Solid Edge part; units mm, degrees
sketch "Sketch1" plane through (0, 0, 0) normal (0, 0, -1) x (-1, 0, 0)
  circle A0 centre (5.5571, -5.7478) radius 2.6503
  line L0 (-56.7501, 0) -> (-56.7501, 10)
  line L1 (-56.7501, 10) -> (67.8618, 10)
  line L2 (67.8618, 0) -> (67.8618, 10)
  line L3 (37.8136, -15.4719) -> (67.8618, 0)
  line L4 (-26.5984, -15.5762) -> (37.8136, -15.4719)
  line L5 (-56.7501, 0) -> (-26.5984, -15.5762)
  circle A1 centre (-19.4469, -5.7778) radius 2.6727
  circle A2 centre (30.5773, -5.7557) radius 2.66
extrude "Protrusion1" add sketch "Sketch1" along normal blind 12
sketch "Sketch2" plane through (56.7501, 5, -6) normal (1, 0, 0) x (0, 0, 1)
  line L0 (-6, -14.1297) -> (-20, 5)
  line L1 (-20, 5) -> (-6, 20.5762)
  line L2 (-6, 20.5762) -> (3.5539, -5)
  line L3 (3.5539, -5) -> (-6, -14.1297)
extrude "ExtrudedCutout_2" cut sketch "Sketch2" along normal mid plane 258
sketch "Sketch3" plane through (0, 0, 0) normal (0, 0, -1) x (-1, 0, 0)
  line L0 (37.8136, -15.4719) -> (67.8618, 0)
  line L1 (67.8618, 0) -> (67.8618, 10)
  line L2 (-56.7501, 10) -> (67.8618, 10)
  line L3 (-56.7501, 0) -> (-56.7501, 10)
  line L4 (-56.7501, 0) -> (-26.5984, -15.5762)
  line L5 (-26.5984, -15.5762) -> (37.8136, -15.4719)
  circle A0 centre (30.5773, -5.7557) radius 2.66
  circle A1 centre (5.5571, -5.7478) radius 2.6503
  circle A2 centre (-19.4469, -5.7778) radius 2.6727
extrude "ExtrudedCutout_3" cut sketch "Sketch3" along normal blind 2.5
Design review of the part built by this model. Coordinates are the model's own, in mm. Coordinates: 2 decimals unless noted, no trailing zeros. Loops run counter-clockwise (first coordinate to the right, second up) from the corner with the lowest first, then second, coordinate; pieces in that order, holes last. Notation, with made-up numbers: (53.5, 41) -> (79.5, 41) arc R24 ccw to (79.5, 75) -> close; hole circle Ø3 at (11.25, -4). An arc over 180 degrees is marked (long way). Use a Markdown table: item, result. Add a question column.
Item 1: Wall thickness on L1, parallel to X at y = -8, z = -4; L2, parallel to Z at x = 31, y = -6; L3, parallel to X at y = -7.75, z = -5.25: over which ranges is each line inside the solid? List them lowest first. Write a range as from..to.
Item 2: We need section C-C, the plane y = -11.25. Write out the cut boundary in (x, z), and give its area (3 significant figures).
Item 3: We need section D-D, the plane z = -10.75. Write out the cut boundary in (x, y).
Item 4: The part is to be moulded in two halves that separate along X. For faces 1 (the flat face through (-5, 0, -2.5)), 2 (the flat face through (38.535, -9.41, -6.128)), 3 (the cylindrical face through (-30.231, -8.393, -5.108)), say which applies: +X half, -X half, draft (parallel to the pull), parting line (faces both ways), or undercut.
Item 5: We need section B-B, the plane z = -4.75. Write out the cut boundary in (x, y).
Item 6: Clearance check with flat-ended pins moving along their axes: P1, Ø10, axis at x = 22, y = 0.5, coming from the -Z side; P2, Ø8.5, axis at x = -5.56, y = -5.75, coming from the -Z side; P3, Ø4, axis at y = -12, z = -6, coming from the +X side. State where each tip first meets the part, or that it passes through.
Item 7: We need section A-A, the plane x = -31.5. Write out the cut boundary in (y, z).
Numbers:
| question | item | result |
|---|---|---|
| 1 | L1 | x = -52.32..-32.01, -29.15..-6.95, -4.16..17.96, 20.93..41.26 |
| 1 | L2 | z = -8.42..-2.5 |
| 1 | L3 | x = -52.81..-32.34, -28.82..-7.29, -3.82..17.64, 21.25..41.75 |
| 2 | outline | (-46.01, -10.38) -> (34.97, -10.38) -> (34.97, -2.5) -> (-46.01, -2.5) -> close |
| 2 | area | 638 mm^2 |
| 3 | outline | (-44.11, -12.23) -> (-37.81, -15.47) -> (26.6, -15.58) -> (33.08, -12.23) -> close |
| 4 | face 1 | draft |
| 4 | face 2 | +X half |
| 4 | face 3 | undercut |
| 5 | outline | (-67.86, 0) -> (-37.81, -15.47) -> (26.6, -15.58) -> (56.75, 0) -> (56.75, 3.83) -> (-67.86, 3.83) -> close; hole circle Ø5.32 at (-30.58, -5.76); hole circle Ø5.3 at (-5.56, -5.75); hole circle Ø5.35 at (19.45, -5.78) |
| 6 | P1 | stops at z = -7.86 |
| 6 | P2 | stops at z = -9.92 |
| 6 | P3 | stops at x = 37.39 |
| 7 | outline | (-15.48, -11.96) -> (-8.25, -9.26) -> (-8.25, -2.5) -> (-15.48, -2.5) -> close; (-3.26, -7.4) -> (9.86, -2.5) -> (-3.26, -2.5) -> close |
